Source: CAD feature listing. Evaluate the final solid. Frame: model axes, mm. Face numbers are marked on the shaded views. A direction names the side the tool comes from. Coordinates: 2 decimals unless noted, no trailing zeros. Order: outer loops, then holes, each group sorted by start corner. A loop starts at its lowest first (then second) coordinate and runs counter-clockwise, first axis right, second up. Notation, with made-up numbers: (30, -9.75) -> (59, -9.75) arc R25 cw to (59, 5.25) -> close; hole circle Ø1 at (11, -38.5). An arc over 180 degrees is marked (long way). Write each question's results on one line, items separated by ' | '. Start each with the question number.
from build123d import *

# Parameters (mm, degrees)
F2_R     = 1.49999
F4_R     = 2.5
F5_DEPTH = 25


# Not quite as in the source:
# - a fillet or chamfer is up to 0.001 mm smaller than in the source, because OpenCascade refuses the exact size


with BuildPart() as f1:
    # F0 (on Front) → F1 (revolve)
    with BuildSketch(Plane.XZ):
        with BuildLine():
            Line((-29.2452627023, 12.6545929811), (-30.7452627023, 12.6545929811))
            Line((-30.7452627023, 12.6545929811), (-30.7452627023, -5.3454070189))
            Line((-30.7452627023, -5.3454070189), (-28.2452627023, -5.3454070189))
            Line((-28.2452627023, -5.3454070189), (-28.2452627023, 6.7686133647))
            Line((-28.2452627023, 6.7686133647), (-29.2452627023, 6.7686133647))
            Line((-29.2452627023, 6.7686133647), (-29.2452627023, 8.7686133647))
            ThreePointArc((-29.2452627023, 8.7686133647), (-29.9124410959, 9.7116031729), (-29.2452627023, 10.6545929811))
            Line((-29.2452627023, 10.6545929811), (-29.2452627023, 12.6545929811))
        make_face()
    revolve(axis=Axis((-22.2452627023, 0, 3.276667092), (0, 0, -1)))

    # F2 (radius 1.5 in the source; OpenCascade refuses exactly that, so slightly less here)
    f2_edges = [f1.edges().sort_by_distance(p)[0] for p in [
        (-13.745263, 0, 12.654593),
    ]]
    fillet(f2_edges, radius=F2_R)

    # F4 (on offset) → F5 (cut)
    with BuildSketch(Plane.YZ.offset(-25)):
        with Locations((0, -4.6502733603)):
            Circle(F4_R)
    extrude(amount=-F5_DEPTH, mode=Mode.SUBTRACT)


solid = f1.part
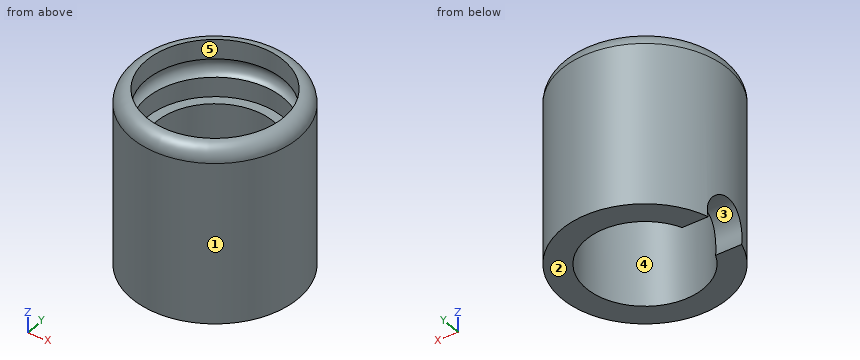
(1) Line query: L1, parallel to Z at x = -27.75, y = 4; L2, parallel to X at y = 4.5, z = 6; L3, parallel to Y at x = -17.75, z = -2.5. Output: solid intervals per line, ascending.
(2) Section C-C on z = -0.75. Return the cut outline in (x, y), then the cut area to 3 significant figures.
(3) First-contact query: P1, Ø4, axis at x = -24, y = -3.5, coming from the +Z side; P2, Ø1, axis at x = -19.5, z = 4.5, coming from the -Y side; P3, Ø6, axis at x = -18.5, z = 3, coming from the +Y side; P4, Ø3, axis at x = -16.5, z = 6.5, coming from the +Y side. Flat tips, straight axial feed; report the tip coordinate or a pass-through.
(4) Reachability of the marked faces 4 and 5 from +Z, -Z, +X, -X, +Y, -Y: full face, straight path, thin tool, end or side. Return the list, or none.
(5) Draft query along Y for the marked faces 1, 2 and 3. Return one class per face: released by +Y, released by -Y, zero draft, split by the parting line, or undercut.
(6) Section B-B on z = 7.25. Return the cut outline in (x, y), then the cut area to 3 significant figures.
Results list:
1) L1: z = -5.35 to 6.77 | L2: x = -29.46 to -26.21, -18.28 to -15.03 | L3: y = -7.21 to -3.97, 3.97 to 7.21
2) outline: circle Ø17 at (-22.25, 0); hole circle Ø12 at (-22.25, 0) | area: 114 mm²
3) P1: passes through | P2: stops at y = -8.2 | P3: stops at y = 8.47 | P4: stops at y = 7.36
4) face 4: +Z, -Z | face 5: +Z
5) face 1: split by the parting line | face 2: zero draft | face 3: undercut
6) outline: circle Ø17 at (-22.25, 0); hole circle Ø14 at (-22.25, 0) | area: 73.0 mm²
